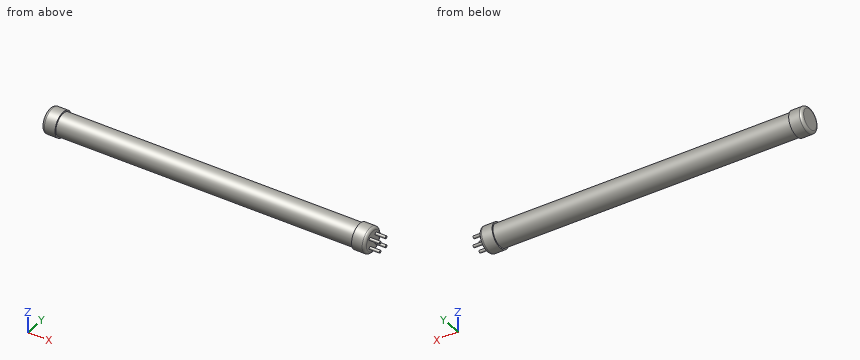
```python
from build123d import *

# Parameters (mm, degrees)
SKETCH1_W           = 224.1
SKETCH1_H           = 8.5
SKETCH2_R           = 9.5
BOSS_EXTRUDE1_DEPTH = 10
FILLET1_R           = 2
SKETCH3_R           = 1
BOSS_EXTRUDE2_DEPTH = 7.7


with BuildPart() as part:
    # Sketch1 → Revolve1 (revolve)
    with BuildSketch(Plane(origin=(0, 0, 0), x_dir=(1, 0, 0), z_dir=(0, 1, 0)), mode=Mode.PRIVATE) as revolve1_sk:
        with Locations((0, 4.25)):
            Rectangle(SKETCH1_W, SKETCH1_H)
    revolve(revolve1_sk.sketch.rotate(Axis((-112.05, 0, 0), (1, 0, 0)), 180), axis=Axis((-112.05, 0, 0), (1, 0, 0)))

    # Sketch2 → Boss-Extrude1 (add)
    with BuildSketch(Plane.ZY.offset(112.05)):
        Circle(SKETCH2_R)
    boss_extrude1 = extrude(amount=BOSS_EXTRUDE1_DEPTH)

    # Mirror1: Boss-Extrude1 across plane
    add(boss_extrude1.mirror(Plane(origin=(0, 0, 0), x_dir=(0, 0, 1), z_dir=(1, 0, 0))))

    # Fillet1
    fillet1_edges = [part.edges().sort_by_distance(p)[0] for p in [
        (122.05, 0, -9.5),
        (-122.05, 0, -9.5),
    ]]
    fillet(fillet1_edges, radius=FILLET1_R)

    # Sketch3 → Boss-Extrude2 (add)
    with BuildSketch(Plane(origin=(122.05, 0, 0), x_dir=(0, 0, -1), z_dir=(1, 0, 0))):
        with Locations(Location((-3.5, 3.5, 0), (0, 0, 180))):
            Circle(SKETCH3_R)
        with Locations(Location((3.5, 3.5, 0), (0, 0, 180))):
            Circle(SKETCH3_R)
        with Locations(Location((3.5, -3.5, 0), (0, 0, 180))):
            Circle(SKETCH3_R)
        with Locations(Location((-3.5, -3.5, 0), (0, 0, 180))):
            Circle(SKETCH3_R)
    extrude(amount=BOSS_EXTRUDE2_DEPTH)


solid = part.part
```
Design review of the part built by this model. Coordinates are the model's own, in mm. Coordinates: 2 decimals unless noted, no trailing zeros. Write each loop counter-clockwise with the first axis right and the second up, starting at its lowest first coordinate (ties: lowest second). Pieces come first, ordered by that corner, then holes.
1) To check wall thickness, follow L1, parallel to X at y = 6, z = 1; L2, parallel to X at y = -8.25, z = 2.5; L3, parallel to X at y = 7.75, z = -5. State the ranges of each line that lie inside material, in increasing order.
2) Insertion check: pin 1 (5 mm diameter, centred on x = -31.5, z = 7, fed in from +Y); pin 2 (4.5 mm diameter, centred on y = -3, z = 0, fed in from +X); pin 3 (10 mm diameter, centred on x = 89, y = 7, fed in from +Z). Each pin has a flat end and moves straight along its axis. Give the tip position at first contact, or say it passes through.
3) Add section A-A (z = 0). Write out the cut boundary in (x, y), plus the area to 3 significant figures.
4) Add section C-C (x = -42). Write out the cut boundary in (y, z), plus the area to 3 significant figures.
Check result:
1. L1: x = -122.05 to 122.05
1. L2: x = -121.71 to -112.05, 112.05 to 121.71
1. L3: x = -121.07 to -112.05, 112.05 to 121.07
2. pin 1: stops at y = 7.21
2. pin 2: stops at x = 122.05
2. pin 3: stops at z = 8.26
3. outline: (-122.05, -7.5) arc R2 ccw to (-120.05, -9.5) - (-112.05, -9.5) - (-112.05, -8.5) - (112.05, -8.5) - (112.05, -9.5) - (120.05, -9.5) arc R2 ccw to (122.05, -7.5) - (122.05, 7.5) arc R2 ccw to (120.05, 9.5) - (112.05, 9.5) - (112.05, 8.5) - (-112.05, 8.5) - (-112.05, 9.5) - (-120.05, 9.5) arc R2 ccw to (-122.05, 7.5) - close
3. area: 4,190 mm2
4. outline: circle Ø17 at (0, 0)
4. area: 227 mm2
